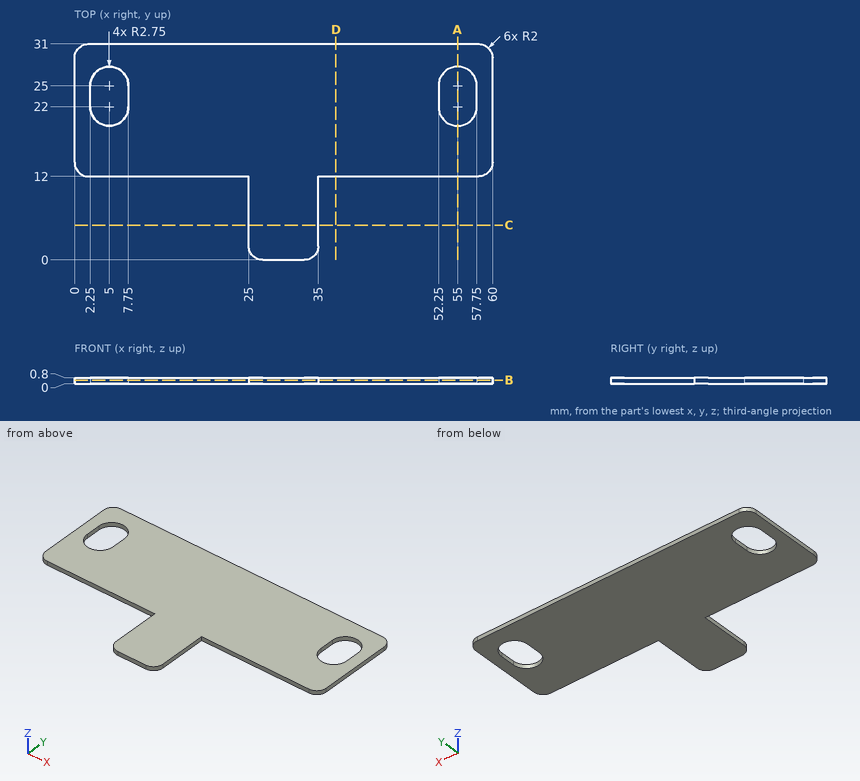
Geometry: see drawing. Coordinates: mm, zero at the bounding-box minimum. Give positions to 0.01 mm unless a question says otherwise; leave off trailing zeros. Write each loop counter-clockwise with the first axis right and the second up, starting at its lowest first coordinate (ties: lowest second). Pieces come first, ordered by that corner, then holes. Notation, with made-up numbers: M -25.75,-0.75 L 14.25,-0.75 A32 cw 14.25,25.25 Z; hole C 62,-23 d5. An arc over 180 degrees is marked long. Return JSON: item names as keys, results as strings. Group by question number.
1) First-contact query: pin 1 Ø3 at (x, y) = (36.5, 19.5) entering from -Z. Flat tip, straight axial feed; report the tip coordinate or a pass-through.
2) Cut plane B-B, the plane z = 0.5. Output: boundary loops of the cut face in (x, y), then the cut area to 3 significant figures.
3) Ray query, L1, parallel to X at y = 25, z = 0.15; L2, parallel to X at y = 26, z = 0.2; L3, parallel to X at y = 3, z = 0.7. Return the intervals inside material, ascending.
4) Cut plane A-A, the plane x = 55. Output: boundary loops of the cut face in (y, z), then the cut area to 3 significant figures.
5) Cut plane D-D, the plane x = 37.5. Output: boundary loops of the cut face in (y, z).
6) Cut plane C-C, the plane y = 5. Output: boundary loops of the cut face in (x, z), then the cut area to 3 significant figures.
Data:
{
 "1": {"pin 1": "stops at z = 0"},
 "2": {"outline": "M 0,14 A2 ccw 2,12 L 25,12 L 25,2 A2 ccw 27,0 L 33,0 A2 ccw 35,2 L 35,12 L 58,12 A2 ccw 60,14 L 60,29 A2 ccw 58,31 L 2,31 A2 ccw 0,29 Z; hole M 2.25,22 A2.75 ccw 7.75,22 L 7.75,25 A2.75 ccw 2.25,25 Z; hole M 52.25,22 A2.75 ccw 57.75,22 L 57.75,25 A2.75 ccw 52.25,25 Z", "area": "1,170 mm²"},
 "3": {"L1": "x = 0 to 2.25, 7.75 to 52.25, 57.75 to 60", "L2": "x = 0 to 2.44, 7.56 to 52.44, 57.56 to 60", "L3": "x = 25 to 35"},
 "4": {"outline": "M 12,0 L 19.25,0 L 19.25,0.8 L 12,0.8 Z; M 27.75,0 L 31,0 L 31,0.8 L 27.75,0.8 Z", "area": "8.40 mm²"},
 "5": {"outline": "M 12,0 L 31,0 L 31,0.8 L 12,0.8 Z"},
 "6": {"outline": "M 25,0 L 35,0 L 35,0.8 L 25,0.8 Z", "area": "8.00 mm²"}
}
